Geometry: final body of the model. Coordinates: model frame, mm. A direction names the side the tool comes from. Coordinates: 2 decimals unless noted, no trailing zeros. Order: outer loops, then holes, each group sorted by start corner. A loop starts at its lowest first (then second) coordinate and runs counter-clockwise, first axis right, second up. Notation, with made-up numbers: M 14,42 L 30,42 A27 ccw 30,69 Z; hole C 27,0 d2. An arc over 180 degrees is marked long. Use CSV: the item, a comma, the result in double quotes. Start each with the question number.
1. Section query D-D on y = 15.5. Return the cut outline in (x, z).
2. First-contact query: P1, Ø6, axis at x = -1, y = 22.5, coming from the -Z side; P2, Ø4, axis at y = 7, z = -1, coming from the +X side (3 decimals); P3, Ø3, axis at x = 0, y = 21.59, coming from the -Z side; P4, Ø2, axis at y = 20, z = 2, coming from the -X side. Flat tips, straight axial feed; report the tip coordinate or a pass-through.
3. Material intervals for line 1 (Y direction, x = -12, z = -1); line 2 (Y direction, x = 0, z = 2.25) (3 decimals); line 3 (X direction, y = -10, z = -4.25) (3 decimals), sorted ascending.
4. Set-up query: faces 4 (the flat face through (34.955, 7, -2)), 5 (the cylindrical face through (-47.24, -5.35, 1.63)), 6 (the flat face through (-40.005, 0, -2)). Return all of +Z, -Z, +X, -X, +Y, -Y with unobstructed straight access to the full face (end or side cutting, diameter ignored); none if empty.
5. Section query C-C on x = -10.5. Return the cut outline in (y, z).
6. Pull-direction query (X, two-part tool) for faces 1 (the cylindrical face through (-5.249, 15.117, 1.628)), 2 (the flat face through (-2.447, -7, -2)), 3 (the flat face through (-1, 2, 3.302)); classes: pulls with the +X half, pulls with the -X half, needs draft (parallel to the pull), parting line crosses it, or undercut.
7. Section query B-B on z = 1. State how many separate pieces and enclosed holes the cut face has, and give its area (3 significant figures).
8. Section query A-A on x = 0. Return the cut outline in (y, z) (3 decimals), and give its area (3 significant figures).
from build123d import *

# Parameters (mm, degrees)
F0_R     = 1.905
F1_DEPTH = 3.302
F3_DEPTH = 4.826
F5_DEPTH = 4.826


with BuildPart() as f1:
    # F0 (on Top) → F1 (new body)
    with BuildSketch(Plane.XY):
        with BuildLine():
            Line((-8.88014, 13.589), (-34.925, 13.589))
            ThreePointArc((-34.925, 13.589), (-38.517102, 12.101102), (-40.005, 8.509))
            Line((-40.005, 8.509), (-40.005, 1.650725))
            Line((-40.005, 1.650725), (-40.005, -12.540665))
            Line((-40.005, -12.540665), (-36.936027, -13.173994))
            ThreePointArc((-36.936027, -13.173994), (-35.951701, -13.484167), (-34.925, -13.589))
            Line((-34.925, -13.589), (34.406297, -13.589))
            ThreePointArc((34.406297, -13.589), (34.922317, -13.562724), (35.432998, -13.484167))
            Line((35.432998, -13.484167), (47.290979, -11.037093))
            ThreePointArc((47.290979, -11.037093), (43.183951, -7.412463), (46.944249, -3.429275))
            Line((46.944249, -3.429275), (45.085, -3.429275))
            ThreePointArc((45.085, -3.429275), (41.492898, -1.941377), (40.005, 1.650725))
            Line((40.005, 1.650725), (40.005, 8.509))
            ThreePointArc((40.005, 8.509), (38.517102, 12.101102), (34.925, 13.589))
            Line((34.925, 13.589), (8.88014, 13.589))
            ThreePointArc((8.88014, 13.589), (5.288038, 15.076898), (3.80014, 18.669))
            Line((3.80014, 18.669), (3.80014, 21.459575))
            ThreePointArc((3.80014, 21.459575), (0, 17.787622), (-3.80014, 21.459575))
            Line((-3.80014, 21.459575), (-3.80014, 18.669))
            ThreePointArc((-3.80014, 18.669), (-5.288038, 15.076898), (-8.88014, 13.589))
        make_face()
        with BuildLine():
            Line((-40.005, -12.540665), (-40.005, 1.650725))
            ThreePointArc((-40.005, 1.650725), (-41.492898, -1.941377), (-45.085, -3.429275))
            Line((-45.085, -3.429275), (-46.944249, -3.429275))
            ThreePointArc((-46.944249, -3.429275), (-44.279796, -4.561147), (-43.18, -7.239))
            ThreePointArc((-43.18, -7.239), (-44.404524, -10.037467), (-47.290979, -11.037093))
            Line((-47.290979, -11.037093), (-40.005, -12.540665))
        make_face()
        with BuildLine():
            Line((-3.80014, 21.720425), (-3.80014, 21.459575))
            ThreePointArc((-3.80014, 21.459575), (0, 17.787622), (3.80014, 21.459575))
            Line((3.80014, 21.459575), (3.80014, 21.720425))
            ThreePointArc((3.80014, 21.720425), (0, 25.392378), (-3.80014, 21.720425))
        make_face()
        with Locations((0, 21.59)):
            Circle(F0_R, mode=Mode.SUBTRACT)
        with BuildLine():
            ThreePointArc((-3.80014, 21.720425), (-3.802378, 21.59), (-3.80014, 21.459575))
            Line((-3.80014, 21.459575), (-3.80014, 21.720425))
        make_face()
        with BuildLine():
            Line((3.80014, 21.720425), (3.80014, 21.459575))
            ThreePointArc((3.80014, 21.459575), (3.801818, 21.524778), (3.802378, 21.59))
            ThreePointArc((3.802378, 21.59), (3.801818, 21.655222), (3.80014, 21.720425))
        make_face()
        with BuildLine():
            Line((-47.035751, -3.429275), (-46.944249, -3.429275))
            ThreePointArc((-46.944249, -3.429275), (-46.99, -3.429), (-47.035751, -3.429275))
        make_face()
        with BuildLine():
            ThreePointArc((-43.18, -7.239), (-44.279796, -4.561147), (-46.944249, -3.429275))
            Line((-46.944249, -3.429275), (-47.035751, -3.429275))
            ThreePointArc((-47.035751, -3.429275), (-50.797858, -7.111254), (-47.290979, -11.037093))
            ThreePointArc((-47.290979, -11.037093), (-44.404524, -10.037467), (-43.18, -7.239))
        make_face()
        with Locations((-46.99, -7.239)):
            Circle(F0_R, mode=Mode.SUBTRACT)
        with BuildLine():
            ThreePointArc((46.944249, -3.429275), (43.183951, -7.412463), (47.290979, -11.037093))
            ThreePointArc((47.290979, -11.037093), (49.788467, -9.824476), (50.8, -7.239))
            ThreePointArc((50.8, -7.239), (49.700204, -4.561147), (47.035751, -3.429275))
            Line((47.035751, -3.429275), (46.944249, -3.429275))
        make_face()
        with Locations((46.99, -7.239)):
            Circle(F0_R, mode=Mode.SUBTRACT)
        with BuildLine():
            ThreePointArc((47.035751, -3.429275), (46.99, -3.429), (46.944249, -3.429275))
            Line((46.944249, -3.429275), (47.035751, -3.429275))
        make_face()
    extrude(amount=F1_DEPTH)

    # F2 (on face) → F3 (join)
    with BuildSketch(Plane(origin=(0, 0, 0), x_dir=(1, 0, 0), z_dir=(0, 0, -1))):
        with BuildLine():
            Line((-40.005, -1.650725), (-40.005, -5.079863))
            Line((-40.005, -5.079863), (-40.005, -8.509))
            ThreePointArc((-40.005, -8.509), (-38.517102, -12.101102), (-34.925, -13.589))
            Line((-34.925, -13.589), (-13.131685, -13.589))
            Line((-13.131685, -13.589), (-8.88014, -13.589))
            Line((-8.88014, -13.589), (8.88014, -13.589))
            Line((8.88014, -13.589), (9.643361, -13.589))
            Line((9.643361, -13.589), (34.925, -13.589))
            ThreePointArc((34.925, -13.589), (38.517102, -12.101102), (40.005, -8.509))
            Line((40.005, -8.509), (40.005, -5.079863))
            Line((40.005, -5.079863), (40.005, -1.650725))
            Line((40.005, -1.650725), (40.005, 12.540665))
            Line((40.005, 12.540665), (35.432998, 13.484167))
            ThreePointArc((35.432998, 13.484167), (34.922317, 13.562724), (34.406297, 13.589))
            Line((34.406297, 13.589), (-34.925, 13.589))
            ThreePointArc((-34.925, 13.589), (-35.951701, 13.484167), (-36.936027, 13.173994))
            Line((-36.936027, 13.173994), (-40.005, 12.540665))
            Line((-40.005, 12.540665), (-40.005, -1.650725))
        make_face()
    extrude(amount=F3_DEPTH)

    # F4 (on face) → F5 (cut)
    with BuildSketch(Plane(origin=(0, 0, -4.826), x_dir=(1, 0, 0), z_dir=(0, 0, -1))):
        with BuildLine():
            ThreePointArc((-34.955431, 4.09772), (-34.583456, 3.199695), (-33.685431, 2.82772))
            Line((-33.685431, 2.82772), (-3.716994, 2.82772))
            ThreePointArc((-3.716994, 2.82772), (-2.818968, 3.199695), (-2.446994, 4.09772))
            Line((-2.446994, 4.09772), (-2.446994, 9.376206))
            ThreePointArc((-2.446994, 9.376206), (-2.818968, 10.274232), (-3.716994, 10.646206))
            Line((-3.716994, 10.646206), (-33.685431, 10.646206))
            ThreePointArc((-33.685431, 10.646206), (-34.583456, 10.274232), (-34.955431, 9.376206))
            Line((-34.955431, 9.376206), (-34.955431, 4.09772))
        make_face()
        with BuildLine():
            ThreePointArc((3.716994, 10.646206), (2.818968, 10.274232), (2.446994, 9.376206))
            Line((2.446994, 9.376206), (2.446994, 4.09772))
            ThreePointArc((2.446994, 4.09772), (2.818968, 3.199695), (3.716994, 2.82772))
            Line((3.716994, 2.82772), (33.685431, 2.82772))
            ThreePointArc((33.685431, 2.82772), (34.583456, 3.199695), (34.955431, 4.09772))
            Line((34.955431, 4.09772), (34.955431, 9.376206))
            ThreePointArc((34.955431, 9.376206), (34.583456, 10.274232), (33.685431, 10.646206))
            Line((33.685431, 10.646206), (3.716994, 10.646206))
        make_face()
        with BuildLine():
            Line((-3.716994, -2.82772), (-33.685431, -2.82772))
            ThreePointArc((-33.685431, -2.82772), (-34.583456, -3.199695), (-34.955431, -4.09772))
            Line((-34.955431, -4.09772), (-34.955431, -9.376206))
            ThreePointArc((-34.955431, -9.376206), (-34.583456, -10.274232), (-33.685431, -10.646206))
            Line((-33.685431, -10.646206), (-3.716994, -10.646206))
            ThreePointArc((-3.716994, -10.646206), (-2.818968, -10.274232), (-2.446994, -9.376206))
            Line((-2.446994, -9.376206), (-2.446994, -4.09772))
            ThreePointArc((-2.446994, -4.09772), (-2.818968, -3.199695), (-3.716994, -2.82772))
        make_face()
        with BuildLine():
            Line((2.446994, -4.09772), (2.446994, -9.376206))
            ThreePointArc((2.446994, -9.376206), (2.818968, -10.274232), (3.716994, -10.646206))
            Line((3.716994, -10.646206), (33.685431, -10.646206))
            ThreePointArc((33.685431, -10.646206), (34.583456, -10.274232), (34.955431, -9.376206))
            Line((34.955431, -9.376206), (34.955431, -4.09772))
            ThreePointArc((34.955431, -4.09772), (34.583456, -3.199695), (33.685431, -2.82772))
            Line((33.685431, -2.82772), (3.716994, -2.82772))
            ThreePointArc((3.716994, -2.82772), (2.818968, -3.199695), (2.446994, -4.09772))
        make_face()
    extrude(amount=-F5_DEPTH, mode=Mode.SUBTRACT)


solid = f1.part
Results list:
1,outline,"M -4.91,0 L 4.91,0 L 4.91,3.3 L -4.91,3.3 Z"
2,P1,"stops at z = 0"
2,P2,"stops at x = 40.005"
2,P3,"passes through"
2,P4,"stops at x = -3.8"
3,line 1,"y = -13.59 to -10.65, -2.83 to 2.83, 10.65 to 13.59"
3,line 2,"y = -13.589 to 19.685, 23.495 to 25.392"
3,line 3,"x = -40.005 to -34.792, -2.611 to 2.611, 34.792 to 40.005"
4,face 4,"-Z"
4,face 5,"+Z, -Z"
4,face 6,"-Z, -X, +Y"
5,outline,"M -13.59,-4.83 L -10.65,-4.83 L -10.65,0 L -2.83,0 L -2.83,-4.83 L 2.83,-4.83 L 2.83,0 L 10.65,0 L 10.65,-4.83 L 13.59,-4.83 L 13.59,3.3 L -13.59,3.3 Z"
6,face 1,"pulls with the -X half"
6,face 2,"undercut"
6,face 3,"needs draft"
7,separate pieces,"1"
7,enclosed holes,"3"
7,area,"2,390 mm²"
8,outline,"M -13.589,-4.826 L 13.589,-4.826 L 13.589,0 L 19.685,0 L 19.685,3.302 L -13.589,3.302 Z; M 23.495,0 L 25.392,0 L 25.392,3.302 L 23.495,3.302 Z"
8,area,"247 mm²"
